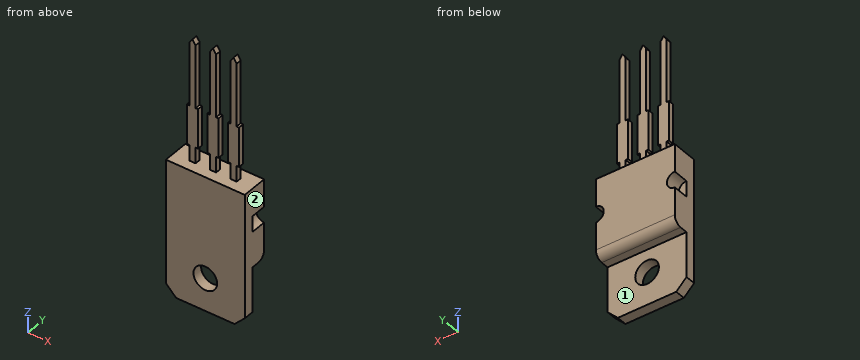
from build123d import *

# Parameters (mm, degrees)
BOSS_EXTRUDE1_DEPTH   = 0.7
BOSS_EXTRUDE1_2_DEPTH = 0.7
BOSS_EXTRUDE1_3_DEPTH = 0.7
SKETCH6_W             = 10
SKETCH6_H             = 10
BOSS_EXTRUDE2_DEPTH   = 2
FILLET1_R             = 1
SKETCH7_R             = 1
CUT_EXTRUDE2_DEPTH    = 2
BOSS_EXTRUDE3_DEPTH   = 1.3
SKETCH9_R             = 1.5
CUT_EXTRUDE3_DEPTH    = 1.3


with BuildPart() as part:
    # Sketch1 → Boss-Extrude1 (new body)
    with BuildSketch(Plane(origin=(0, 0, 0), x_dir=(1, 0, 0), z_dir=(0, 1, 0))):
        Polygon((0, 0), (0.4, -0.594509979), (0.8, 0), (0.8, 7.984975303), (1.1, 7.984975303), (1.1, 13), (0.8, 13), (0.8, 15), (0, 15), (0, 13), (-0.3, 13), (-0.3, 7.984975303), (0, 7.984975303), align=None)
    extrude(amount=BOSS_EXTRUDE1_DEPTH)



with BuildPart() as body_2:
    # Sketch1 → Boss-Extrude1 2 (new body)
    with BuildSketch(Plane(origin=(0, 0, 0), x_dir=(1, 0, 0), z_dir=(0, 1, 0))):
        Polygon((-2.6, 7.984975303), (-2.9, 7.984975303), (-2.9, 13), (-2.6, 13), (-2.6, 15), (-1.8, 15), (-1.8, 13), (-1.5, 13), (-1.5, 7.984975303), (-1.8, 7.984975303), (-1.8, 0), (-2.2, -0.594509979), (-2.6, 0), align=None)
    extrude(amount=BOSS_EXTRUDE1_2_DEPTH)


with BuildPart() as body_3:
    # Sketch1 → Boss-Extrude1 3 (new body)
    with BuildSketch(Plane(origin=(0, 0, 0), x_dir=(1, 0, 0), z_dir=(0, 1, 0))):
        Polygon((-5.2, 0), (-4.8, -0.594509979), (-4.4, 0), (-4.4, 7.984975303), (-4.1, 7.984975303), (-4.1, 13), (-4.4, 13), (-4.4, 15), (-5.2, 15), (-5.2, 13), (-5.5, 13), (-5.5, 7.984975303), (-5.2, 7.984975303), align=None)
    extrude(amount=BOSS_EXTRUDE1_3_DEPTH)


with BuildPart() as part_1:
    add(part.part)

    add(body_2.part)  # Boss-Extrude2 merges body 2

    add(body_3.part)  # Boss-Extrude2 merges body 3
    # Sketch6 → Boss-Extrude2 (add)
    with BuildSketch(Plane(origin=(0, 0, 0), x_dir=(1, 0, 0), z_dir=(0, 1, 0))):
        with Locations((-2.2, 20)):
            Rectangle(SKETCH6_W, SKETCH6_H)
    extrude(amount=BOSS_EXTRUDE2_DEPTH)

    # Fillet1
    fillet1_edges = [part_1.edges().sort_by_distance(p)[0] for p in [
        (-2.2, 2, -25),
    ]]
    fillet(fillet1_edges, radius=FILLET1_R)

    # Sketch7 → Cut-Extrude2 (cut)
    with BuildSketch(Plane(origin=(0, 2, 0), x_dir=(1, 0, 0), z_dir=(0, 1, 0))):
        with Locations((-7.2, 19.5)):
            Circle(SKETCH7_R)
        with Locations((2.8, 19.5)):
            Circle(SKETCH7_R)
    extrude(amount=-CUT_EXTRUDE2_DEPTH, mode=Mode.SUBTRACT)

    # Sketch8 → Boss-Extrude3 (add)
    with BuildSketch(Plane.XZ):
        Polygon((-7.2, -15), (2.8, -15), (2.8, -30.7), (1.5, -32), (-5.9, -32), (-7.2, -30.7), align=None)
    extrude(amount=BOSS_EXTRUDE3_DEPTH)

    # Sketch9 → Cut-Extrude3 (cut)
    with BuildSketch(Plane(origin=(0, 0, 0), x_dir=(1, 0, 0), z_dir=(0, 1, 0))):
        with Locations(Location((-2.2, 27.85, 0), (0, 0, 270))):
            Circle(SKETCH9_R)
    extrude(amount=-CUT_EXTRUDE3_DEPTH, mode=Mode.SUBTRACT)


solid = part_1.part
The listing builds one solid part. Answer for the finished solid, in the listing's coordinates (mm). Face numbers are marked on the shaded views. A direction names the side the tool comes from. Give positions to 0.01 mm unless a question says otherwise; leave off trailing zeros. Order: outer loops, then holes, each group sorted by start corner. A loop starts at its lowest first (then second) coordinate and runs counter-clockwise, first axis right, second up. Notation, with made-up numbers: (-3.5, 32.5) - (39.5, 32.5) arc R14 ccw to (39.5, 41.5) - close; hole circle Ø8 at (58, -35.75). An arc over 180 degrees is marked (long way). Use one line per item in the form item = value.
1) Find section D-D on y = 1.5. Determine the outline of the cut face in (x, z), and give its area (3 significant figures).
Verdict:
outline = (-7.2, -24.87) - (2.8, -24.87) - (2.8, -20.5) arc R1 cw to (2.8, -18.5) - (2.8, -15) - (-7.2, -15) - (-7.2, -18.5) arc R1 cw to (-7.2, -20.5) - close
area = 95.5 mm^2
2) Each of these flat-tipped pins is pushed along its axis until it touches: pin 1 (0.8 mm diameter, centred on y = 0.5, z = -11.5, fed in from +X); pin 2 (0.5 mm diameter, centred on x = -0.5, y = 0.5, fed in from -Z); pin 3 (0.5 mm diameter, centred on x = -7, z = -20, fed in from +Y). Where does it stop, or does it pass through?
Verdict:
pin_1 = 1.1
pin_2 = -25
pin_3 = 0
3) Find section B-B on z = -27.85. Determine the outline of the cut face in (x, y), and give its area (3 significant figures).
Verdict:
outline = (-7.2, -1.3) - (-3.7, -1.3) - (-3.7, 0) - (-7.2, 0) - close; (-0.7, -1.3) - (2.8, -1.3) - (2.8, 0) - (-0.7, 0) - close
area = 9.10 mm^2
4) For the marked faces 1 and 2, determine the directions among +Z, -Z, +X, -X, +Y, -Y from which every point of the face is accessible in a straight line to the end or side of a thin tool.
Verdict:
face_1 = -Z, +X, -X, +Y
face_2 = +Z, -Z, +X, +Y, -Y
5) Find section A-A on z = -14.5. Determine the outline of the cut face in (x, y), and give its area (3 significant figures).
Verdict:
outline = (-5.2, 0) - (-4.4, 0) - (-4.4, 0.7) - (-5.2, 0.7) - close; (-2.6, 0) - (-1.8, 0) - (-1.8, 0.7) - (-2.6, 0.7) - close; (0, 0) - (0.8, 0) - (0.8, 0.7) - (0, 0.7) - close
area = 1.68 mm^2
6) Find section C-C on z = -19.5. Determine the outline of the cut face in (x, y).
Verdict:
outline = (-7.2, -1.3) - (2.8, -1.3) - (2.8, 0) - (1.8, 0) - (1.8, 2) - (-6.2, 2) - (-6.2, 0) - (-7.2, 0) - close
7) Consider probe 1 along X at (y, z) = (-0.8, -27.85); probe 2 along Y at (x, z) = (2.5, -29); probe 3 along Z at (x, y) = (1, 1.05). Determine where each line is inside the solid, lowest interval first. Write a range as [from, to].
Verdict:
probe_1 = [-7.2, -3.7], [-0.7, 2.8]
probe_2 = [-1.3, 0]
probe_3 = [-25, -15]
